Part model, mm, in its own coordinate system. Face numbers are marked on the shaded views. A direction names the side the tool comes from. Give positions to 0.01 mm unless a question says otherwise; leave off trailing zeros. Order: outer loops, then holes, each group sorted by start corner. A loop starts at its lowest first (then second) coordinate and runs counter-clockwise, first axis right, second up. Notation, with made-up numbers: M -37,29.25 L -1,29.25 A24 ccw -1,64.25 Z; hole C 3.5,52.5 d3. An arc over 180 degrees is marked long. Return JSON: item names as keys, results as strings.
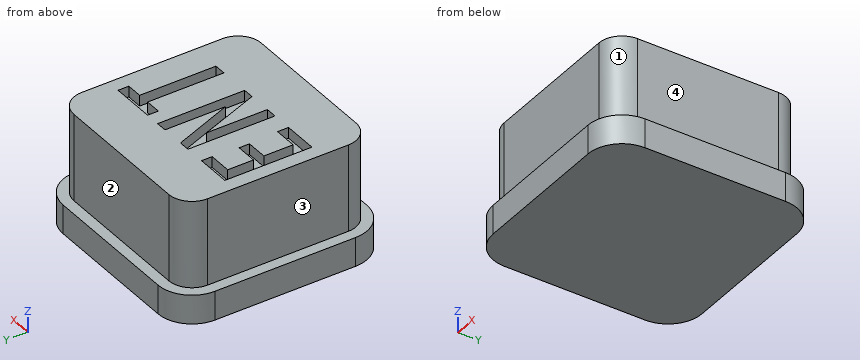
from build123d import *

# Parameters (mm, degrees)
F1_DEPTH = 2
F2_DEPTH = 8
F3_DEPTH = 7.25


with BuildPart() as f1:
    # F0 (on Top) → F1 (new body)
    with BuildSketch(Plane.XY):
        with BuildLine():
            Line((4.85, 7.2), (-4.85, 7.2))
            ThreePointArc((-4.85, 7.2), (-6.511701, 6.511701), (-7.2, 4.85))
            Line((-7.2, 4.85), (-7.2, -4.85))
            ThreePointArc((-7.2, -4.85), (-6.511701, -6.511701), (-4.85, -7.2))
            Line((-4.85, -7.2), (4.85, -7.2))
            ThreePointArc((4.85, -7.2), (6.511701, -6.511701), (7.2, -4.85))
            Line((7.2, -4.85), (7.2, 4.85))
            ThreePointArc((7.2, 4.85), (6.511701, 6.511701), (4.85, 7.2))
        make_face()
        with BuildLine():
            ThreePointArc((6.45, -4.85), (5.981371, -5.981371), (4.85, -6.45))
            Line((4.85, -6.45), (-4.85, -6.45))
            ThreePointArc((-4.85, -6.45), (-5.981371, -5.981371), (-6.45, -4.85))
            Line((-6.45, -4.85), (-6.45, 4.85))
            ThreePointArc((-6.45, 4.85), (-5.981371, 5.981371), (-4.85, 6.45))
            Line((-4.85, 6.45), (4.85, 6.45))
            ThreePointArc((4.85, 6.45), (5.981371, 5.981371), (6.45, 4.85))
            Line((6.45, 4.85), (6.45, -4.85))
        make_face(mode=Mode.SUBTRACT)
    extrude(amount=F1_DEPTH)

    # F0 (on Top) → F2 (join)
    with BuildSketch(Plane.XY):
        with BuildLine():
            Line((-4.85, -6.45), (4.85, -6.45))
            ThreePointArc((4.85, -6.45), (5.981371, -5.981371), (6.45, -4.85))
            Line((6.45, -4.85), (6.45, 4.85))
            ThreePointArc((6.45, 4.85), (5.981371, 5.981371), (4.85, 6.45))
            Line((4.85, 6.45), (-4.85, 6.45))
            ThreePointArc((-4.85, 6.45), (-5.981371, 5.981371), (-6.45, 4.85))
            Line((-6.45, 4.85), (-6.45, -4.85))
            ThreePointArc((-6.45, -4.85), (-5.981371, -5.981371), (-4.85, -6.45))
        make_face()
        Polygon((-3.077863, -3), (-5.468703, -3), (-5.468703, 3), (-3.077863, 3), (-3.077863, 2.267176), (-4.671756, 2.267176), (-4.671756, 0.490077), (-3.196947, 0.490077), (-3.196947, -0.224427), (-4.671756, -0.224427), (-4.671756, -2.239694), (-3.077863, -2.239694), align=None, mode=Mode.SUBTRACT)
        Polygon((-0.906871, -3), (-1.685497, -3), (-1.685497, 3), (-0.925191, 3), (0.668702, -1.158778), (0.668702, 3), (1.419847, 3), (1.419847, -3), (0.668702, -3), (-0.906871, 1.204581), align=None, mode=Mode.SUBTRACT)
        Polygon((4.360305, -3), (3.545038, -3), (3.545038, 2.258016), (2.445801, 2.258016), (2.445801, 3), (5.468702, 3), (5.468702, 2.258016), (4.360305, 2.258016), align=None, mode=Mode.SUBTRACT)
    extrude(amount=F2_DEPTH)

    # F0 (on Top) → F3 (join)
    with BuildSketch(Plane.XY):
        Polygon((-5.468703, 3), (-5.468703, -3), (-3.077863, -3), (-3.077863, -2.239694), (-4.671756, -2.239694), (-4.671756, -0.224427), (-3.196947, -0.224427), (-3.196947, 0.490077), (-4.671756, 0.490077), (-4.671756, 2.267176), (-3.077863, 2.267176), (-3.077863, 3), align=None)
        Polygon((-1.685497, 3), (-1.685497, -3), (-0.906871, -3), (-0.906871, 1.204581), (0.668702, -3), (1.419847, -3), (1.419847, 3), (0.668702, 3), (0.668702, -1.158778), (-0.925191, 3), align=None)
        Polygon((3.545038, 2.258016), (3.545038, -3), (4.360305, -3), (4.360305, 2.258016), (5.468702, 2.258016), (5.468702, 3), (2.445801, 3), (2.445801, 2.258016), align=None)
    extrude(amount=F3_DEPTH)


solid = f1.part
Q1. Band-saw the part on B-B (y = -2). Give the cut face in (x, z), then the cut area to 3 significant figures.
Established:
{"outline": "M -7.2,0 L 7.2,0 L 7.2,2 L 6.45,2 L 6.45,8 L 4.36,8 L 4.36,7.25 L 3.55,7.25 L 3.55,8 L 1.42,8 L 1.42,7.25 L 0.29,7.25 L 0.29,8 L -0.91,8 L -0.91,7.25 L -1.69,7.25 L -1.69,8 L -4.67,8 L -4.67,7.25 L -5.47,7.25 L -5.47,8 L -6.45,8 L -6.45,2 L -7.2,2 Z", "area": "104 mm²"}
Q2. Band-saw the part on A-A (z = 1.75). Give the cut face in (x, y), then the cut area to 3 significant figures.
Established:
{"outline": "M -7.2,-4.85 A2.35 ccw -4.85,-7.2 L 4.85,-7.2 A2.35 ccw 7.2,-4.85 L 7.2,4.85 A2.35 ccw 4.85,7.2 L -4.85,7.2 A2.35 ccw -7.2,4.85 Z", "area": "203 mm²"}
Q3. Band-saw the part on D-D (x = -1.5). Give the cut face in (y, z).
Established:
{"outline": "M -7.2,0 L 7.2,0 L 7.2,2 L 6.45,2 L 6.45,8 L 3,8 L 3,7.25 L -3,7.25 L -3,8 L -6.45,8 L -6.45,2 L -7.2,2 Z"}
Q4. Probe line 1 along X through (y, z) = (-1.5, 7.75); line 2 along X through (y, z) = (-1.25, 6.5). List the from-to ranges inside material, lowest first.
Established:
{"line 1": "x = -6.45 to -5.47, -4.67 to -1.69, -0.91 to 0.11, 1.42 to 3.55, 4.36 to 6.45", "line 2": "x = -6.45 to 6.45"}
Q5. Band-saw the part on C-C (x = -4). Give the cut face in (y, z), then the cut area to 3 significant figures.
Established:
{"outline": "M -7.2,0 L 7.2,0 L 7.2,2 L 6.45,2 L 6.45,8 L 3,8 L 3,7.25 L 2.27,7.25 L 2.27,8 L 0.49,8 L 0.49,7.25 L -0.22,7.25 L -0.22,8 L -2.24,8 L -2.24,7.25 L -3,7.25 L -3,8 L -6.45,8 L -6.45,2 L -7.2,2 Z", "area": "105 mm²"}
Q6. 3-axis set-ups, long thin cutter, end or side, ignore diameter. For the marked faces 1, 2, 3 and 4: which of +Z, -Z, +X, -X, +Y, -Y reach the whole face in a straight line?
Established:
{"face 1": "+Z, +X, -Y", "face 2": "+Z, +X, -X, +Y", "face 3": "+Z, -X, +Y, -Y", "face 4": "+Z, +X, +Y, -Y"}
Q7. Pin check, flat tips, straight feed: pin 1 (1.5 mm diameter, centred on y = -4.5, z = 3.5, fed in from -X); pin 2 (0.8 mm diameter, centred on x = -4, z = 7.5, fed in from -Y); pin 3 (0.6 mm diameter, centred on x = 1, z = 8, fed in from +Y). Stop position of each tip, or through.
Established:
{"pin 1": "stops at x = -6.45", "pin 2": "stops at y = -6.45", "pin 3": "stops at y = 6.45"}
